from build123d import *

# Parameters (mm, degrees)
SKETCH1_R           = 2.38125
SKETCH1_R_2         = 12.413
SKETCH1_R_3         = 2.413
BOSS_EXTRUDE1_DEPTH = 3.175
FILLET1_R           = 10


with BuildPart() as part:
    # Sketch1 → Boss-Extrude1 (new body)
    with BuildSketch(Plane(origin=(0, 0, 0), x_dir=(1, 0, 0), z_dir=(0, 1, 0))):
        with BuildLine():
            ThreePointArc((-8.046041628, -19.942425209), (-11.245341357, -24.172368354), (-12.38125, -29.352875022))
            ThreePointArc((-12.38125, -29.352875022), (0, -41.734125022), (12.38125, -29.352875022))
            ThreePointArc((12.38125, -29.352875022), (11.245341357, -24.172368354), (8.046041628, -19.942425209))
            add(Edge.make_bspline(
                [(-8.046041628, -19.942425209), (-7.058484548, -20.785974262), (-4.539606647, -22.332996604), (0, -23.235965205), (4.539606647, -22.332996604), (7.058484548, -20.785974262), (8.046041628, -19.942425209)],
                knots=[4.00497242, 4.00497242, 4.00497242, 4.00497242, 4.319689899, 4.71238898, 5.105088062, 5.419805541, 5.419805541, 5.419805541, 5.419805541], degree=3))
        make_face()
        with Locations((0, -29.352875022)):
            Circle(SKETCH1_R, mode=Mode.SUBTRACT)
        with BuildLine():
            Line((-12.38125, -10.532423695), (-12.38125, -29.352875022))
            ThreePointArc((-12.38125, -29.352875022), (-11.245341357, -24.172368354), (-8.046041628, -19.942425209))
            add(Edge.make_bspline(
                [(-12.38125, -10.532423695), (-12.38125, -10.937602676), (-12.301779915, -12.5583186), (-11.507079063, -15.737360854), (-9.718393414, -18.414272732), (-8.290741365, -19.733408195), (-8.046041628, -19.942425209)],
                knots=[3.141592654, 3.141592654, 3.141592654, 3.141592654, 3.239767424, 3.534291735, 3.926990817, 4.00497242, 4.00497242, 4.00497242, 4.00497242], degree=3))
        make_face()
        with BuildLine():
            ThreePointArc((8.046041628, -19.942425209), (0, -16.971625022), (-8.046041628, -19.942425209))
            add(Edge.make_bspline(
                [(-8.046041628, -19.942425209), (-7.058484548, -20.785974262), (-4.539606647, -22.332996604), (0, -23.235965205), (4.539606647, -22.332996604), (7.058484548, -20.785974262), (8.046041628, -19.942425209)],
                knots=[4.00497242, 4.00497242, 4.00497242, 4.00497242, 4.319689899, 4.71238898, 5.105088062, 5.419805541, 5.419805541, 5.419805541, 5.419805541], degree=3))
        make_face()
        with BuildLine():
            ThreePointArc((8.046041628, -19.942425209), (11.245341357, -24.172368354), (12.38125, -29.352875022))
            Line((12.38125, -29.352875022), (12.38125, -10.532423695))
            add(Edge.make_bspline(
                [(8.046041628, -19.942425209), (8.290741365, -19.733408195), (9.718393414, -18.414272732), (11.736565023, -15.393916665), (12.38125, -12.152921351), (12.38125, -10.532423695)],
                knots=[5.419805541, 5.419805541, 5.419805541, 5.419805541, 5.497787144, 5.890486225, 6.283185307, 6.283185307, 6.283185307, 6.283185307], degree=3))
        make_face()
        with BuildLine():
            add(Edge.make_bspline(
                [(12.38125, -10.532423695), (12.38125, -8.911926038), (11.736565023, -5.670930724), (8.982733505, -1.549600459), (4.861396275, 1.204142363), (0, 2.171117815), (-4.861396275, 1.204142363), (-8.982733505, -1.549600459), (-11.507079063, -5.327486536), (-12.301779915, -8.506528789), (-12.38125, -10.127244714), (-12.38125, -10.532423695)],
                knots=[0, 0, 0, 0, 0.392699082, 0.785398163, 1.178097245, 1.570796327, 1.963495408, 2.35619449, 2.748893572, 3.043417883, 3.141592654, 3.141592654, 3.141592654, 3.141592654], degree=3))
            add(Edge.make_bspline(
                [(-12.38125, -10.532423695), (-12.38125, -10.937602676), (-12.301779915, -12.5583186), (-11.507079063, -15.737360854), (-9.718393414, -18.414272732), (-8.290741365, -19.733408195), (-8.046041628, -19.942425209)],
                knots=[3.141592654, 3.141592654, 3.141592654, 3.141592654, 3.239767424, 3.534291735, 3.926990817, 4.00497242, 4.00497242, 4.00497242, 4.00497242], degree=3))
            ThreePointArc((-8.046041628, -19.942425209), (0, -16.971625022), (8.046041628, -19.942425209))
            add(Edge.make_bspline(
                [(8.046041628, -19.942425209), (8.290741365, -19.733408195), (9.718393414, -18.414272732), (11.736565023, -15.393916665), (12.38125, -12.152921351), (12.38125, -10.532423695)],
                knots=[5.419805541, 5.419805541, 5.419805541, 5.419805541, 5.497787144, 5.890486225, 6.283185307, 6.283185307, 6.283185307, 6.283185307], degree=3))
        make_face()
        with BuildLine():
            add(Edge.make_bspline(
                [(2.38125, -10.532423695), (2.38125, -6.408035977), (-1.190625, -8.470229836), (-4.7625, -10.532423695), (-1.190625, -12.594617554), (2.38125, -14.656811413), (2.38125, -10.532423695)],
                knots=[0, 0, 0, 2.094395102, 2.094395102, 4.188790205, 4.188790205, 6.283185307, 6.283185307, 6.283185307], degree=2, weights=[1, 0.5, 1, 0.5, 1, 0.5, 1]))
        make_face(mode=Mode.SUBTRACT)
        with BuildLine():
            Line((-31.105374648, 23.312068051), (-12.38125, -10.532423695))
            add(Edge.make_bspline(
                [(12.38125, -10.532423695), (12.38125, -8.911926038), (11.736565023, -5.670930724), (8.982733505, -1.549600459), (4.861396275, 1.204142363), (0, 2.171117815), (-4.861396275, 1.204142363), (-8.982733505, -1.549600459), (-11.507079063, -5.327486536), (-12.301779915, -8.506528789), (-12.38125, -10.127244714), (-12.38125, -10.532423695)],
                knots=[0, 0, 0, 0, 0.392699082, 0.785398163, 1.178097245, 1.570796327, 1.963495408, 2.35619449, 2.748893572, 3.043417883, 3.141592654, 3.141592654, 3.141592654, 3.141592654], degree=3))
            Line((12.38125, -10.532423695), (31.105374628, 23.312068057))
            ThreePointArc((31.105374628, 23.312068057), (9.550975447, 23.016676344), (20.2438, 41.734124978))
            Line((20.2438, 41.734124978), (-20.2438, 41.734124978))
            ThreePointArc((-20.2438, 41.734124978), (-11.466483525, 38.098441453), (-7.8308, 29.321124978))
            ThreePointArc((-7.8308, 29.321124978), (-17.140749655, 17.302237861), (-31.105374648, 23.312068051))
        make_face()
        with Locations((20.243799976, 29.321124978)):
            Circle(SKETCH1_R_2)
        with Locations((20.2438, 29.321125022)):
            Circle(SKETCH1_R_3, mode=Mode.SUBTRACT)
        with Locations((-20.2438, 29.321124978)):
            Circle(SKETCH1_R_2)
        with Locations((-20.2438, 29.321124978)):
            Circle(SKETCH1_R_3, mode=Mode.SUBTRACT)
    extrude(amount=BOSS_EXTRUDE1_DEPTH)

    # Fillet1
    fillet1_edges = [part.edges().sort_by_distance(p)[0] for p in [
        (-12.38125, 1.5875, 10.532423695),
        (12.38125, 1.5875, 10.532423695),
    ]]
    fillet(fillet1_edges, radius=FILLET1_R)


solid = part.part
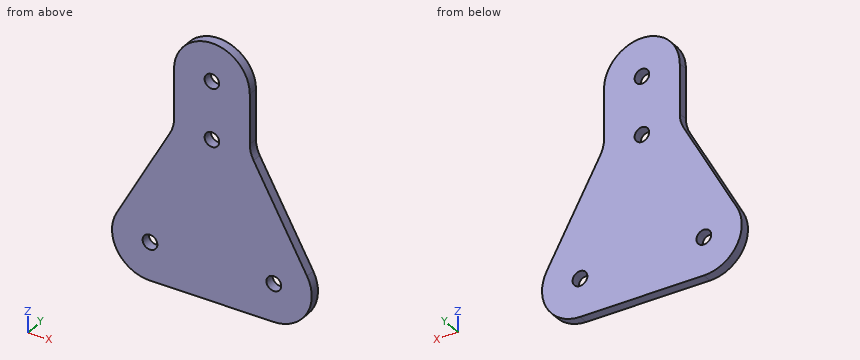
Geometry check sheet. Reference: the model listing, model coordinates, mm. Coordinates: 2 decimals unless noted, no trailing zeros. Loops run counter-clockwise (first coordinate to the right, second up) from the corner with the lowest first, then second, coordinate; pieces in that order, holes last. Notation, with made-up numbers: (-7, 26) - (42, 26) arc R27 ccw to (42, 48) - close; hole circle Ø9 at (67.5, 35.5). An arc over 180 degrees is marked (long way). Use one line per item in the form item = value. Start each with the question number.
Item 1: Section check A-A, the plane x = 0. Give the number of separate pieces and of enclosed holes in the cut face, and give its area (3 significant figures).
Item 2: Thickness scan on probe 1 along Z at (x, y) = (0, 1.8); probe 2 along X at (y, z) = (2.8, -29); probe 3 along Z at (x, y) = (-1, 2.4). Record the ranges inside material, lowest first.
Item 3: Gauge pin test, flat ends, axial feed: pin 1 (1.6 mm diameter, centred on y = 2, z = 25, fed in from -X); pin 2 (3 mm diameter, centred on x = 0, z = 29.35, fed in from +Y); pin 3 (1 mm diameter, centred on y = 0.5, z = 27.5, fed in from +X); pin 4 (1 mm diameter, centred on y = 1, z = -1.5, fed in from -X). Record the tip position at first contact, or that the pin passes through.
Item 4: Section check B-B, the plane z = 35. Enter the section's corners in (x, y) (3 decimals).
Item 5: Section check D-D, the plane x = 7. Enter the section's corners in (y, z) (3 decimals), and give its area (3 significant figures).
Computed:
q1.separate_pieces = 3
q1.enclosed_holes = 0
q1.area = 235 mm2
q2.probe_1 = -41.73 to 8.15, 12.91 to 26.97, 31.73 to 41.73
q2.probe_2 = -32.65 to -22.64, -17.85 to 17.85, 22.64 to 32.65
q2.probe_3 = -41.73 to 8.37, 12.69 to 27.19, 31.51 to 41.69
q3.pin_1 = -12.38
q3.pin_2 = through
q3.pin_3 = 12.38
q3.pin_4 = -19.31
q4.outline = (-11.018, 0) - (11.018, 0) - (11.018, 3.175) - (-11.018, 3.175) - close
q5.outline = (0, -41.734) - (3.175, -41.734) - (3.175, 39.565) - (0, 39.565) - close
q5.area = 258 mm2
